Job drawing, mm, ordinate dimensions from the low corner. One solid piece. A direction names the side the tool comes from. Give positions to 0.01 mm unless a question says otherwise; leave off trailing zeros. Write each loop counter-clockwise with the first axis right and the second up, starting at its lowest first coordinate (ties: lowest second). Pieces come first, ordered by that corner, then holes. Notation, with made-up numbers: (44, 42.5) - (54, 42.5) arc R7 ccw to (54, 50.5) - close; hole circle Ø2 at (44.25, 74). An arc over 180 degrees is marked (long way). Answer in a Markdown table with one row per item. Add a question column.
1. Band-saw the part on A-A on y = 5.25. Write the cut outline in (x, z).
2. Probe line 1 along X through (y, z) = (7.5, 1.75); line 2 along X through (y, z) = (7.3, 17.5); line 3 along Z through (x, y) = (21.5, 3.75). List the from-to ranges inside material, lowest first.
3. Which spindle directions (+Z, -Z, +X, -X, +Y, -Y) get a long thin tool onto all of the face, cutting with end or side? Do the marked faces 1, 2 and 3. Say none if no direction does.
4. Pull direction X, two halves, no side cores. Call the marked faces 4, 5, 6 and 7: released by +X, released by -X, zero draft, split by the parting line, or undercut.
5. Band-saw the part on C-C on x = 17. Write the cut outline in (y, z), plus the area to 3 significant figures.
6. Band-saw the part on D-D on x = 14. Write the cut outline in (y, z), plus the area to 3 significant figures.
7. Band-saw the part on B-B on z = 6. Write the cut outline in (x, y).
8. Drop flat-ended pins along their axis: pin 1 Ø3 at (y, z) = (6, 11) entering from -X; pin 2 Ø1.4 at (x, z) = (26.25, 1.75) entering from +Y; pin 3 Ø11 at (x, z) = (11.5, 11) entering from +Y. Give the stop position or say it passes through.
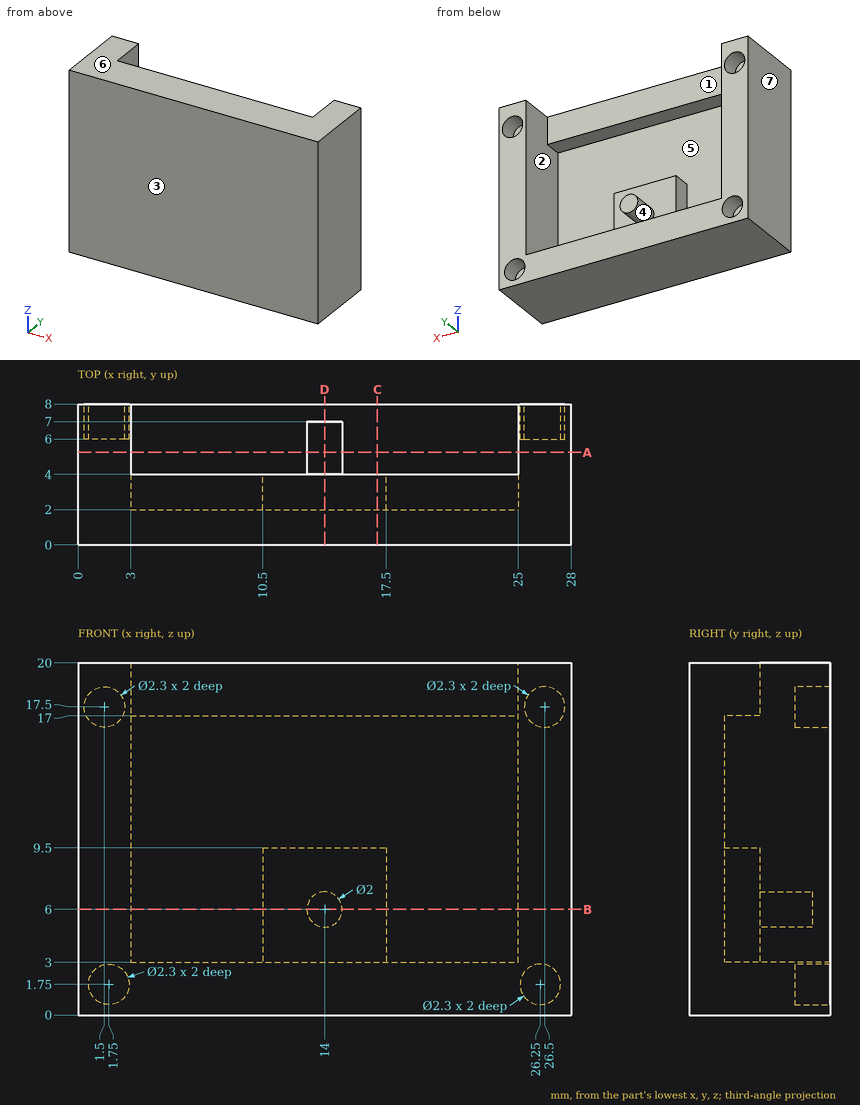
Values:
| question | item | result |
|---|---|---|
| 1 | outline | (0, 0) - (28, 0) - (28, 20) - (25, 20) - (25, 3) - (3, 3) - (3, 20) - (0, 20) - close; circle Ø2 at (14, 6) |
| 2 | line 1 | x = 0 to 0.6, 2.9 to 25.1, 27.4 to 28 |
| 2 | line 2 | x = 0 to 0.35, 2.65 to 3, 25 to 25.35, 27.65 to 28 |
| 2 | line 3 | z = 0 to 3, 17 to 20 |
| 3 | face 1 | +Z, +Y |
| 3 | face 2 | +Y |
| 3 | face 3 | +Z, -Z, +X, -X, -Y |
| 4 | face 4 | undercut |
| 4 | face 5 | undercut |
| 4 | face 6 | zero draft |
| 4 | face 7 | released by -X |
| 5 | outline | (0, 0) - (8, 0) - (8, 3) - (4, 3) - (4, 9.5) - (2, 9.5) - (2, 17) - (4, 17) - (4, 20) - (0, 20) - close |
| 5 | area | 77.0 mm² |
| 6 | outline | (0, 0) - (8, 0) - (8, 3) - (4, 3) - (4, 5) - (7, 5) - (7, 7) - (4, 7) - (4, 9.5) - (2, 9.5) - (2, 17) - (4, 17) - (4, 20) - (0, 20) - close |
| 6 | area | 83.0 mm² |
| 7 | outline | (0, 0) - (28, 0) - (28, 8) - (25, 8) - (25, 2) - (17.5, 2) - (17.5, 4) - (15, 4) - (15, 7) - (13, 7) - (13, 4) - (10.5, 4) - (10.5, 2) - (3, 2) - (3, 8) - (0, 8) - close |
| 8 | pin 1 | stops at x = 0 |
| 8 | pin 2 | stops at y = 6 |
| 8 | pin 3 | stops at y = 7 |
